Source: three-view drawing plus pictorial views. Frame: mm from the lowest corner of the part. A direction names the side the tool comes from. Round coordinates to 2 decimals unless told otherwise and drop trailing zeros. Write each loop counter-clockwise with the first axis right and the second up, starting at its lowest first coordinate (ties: lowest second). Pieces come first, ordered by that corner, then holes. Notation, with made-up numbers: (64, 75) -> (101, 75) arc R7 cw to (101, 82) -> close; hole circle Ø10 at (69, -3.75). An arc over 180 degrees is marked (long way). Put each result on its own line as item: value.
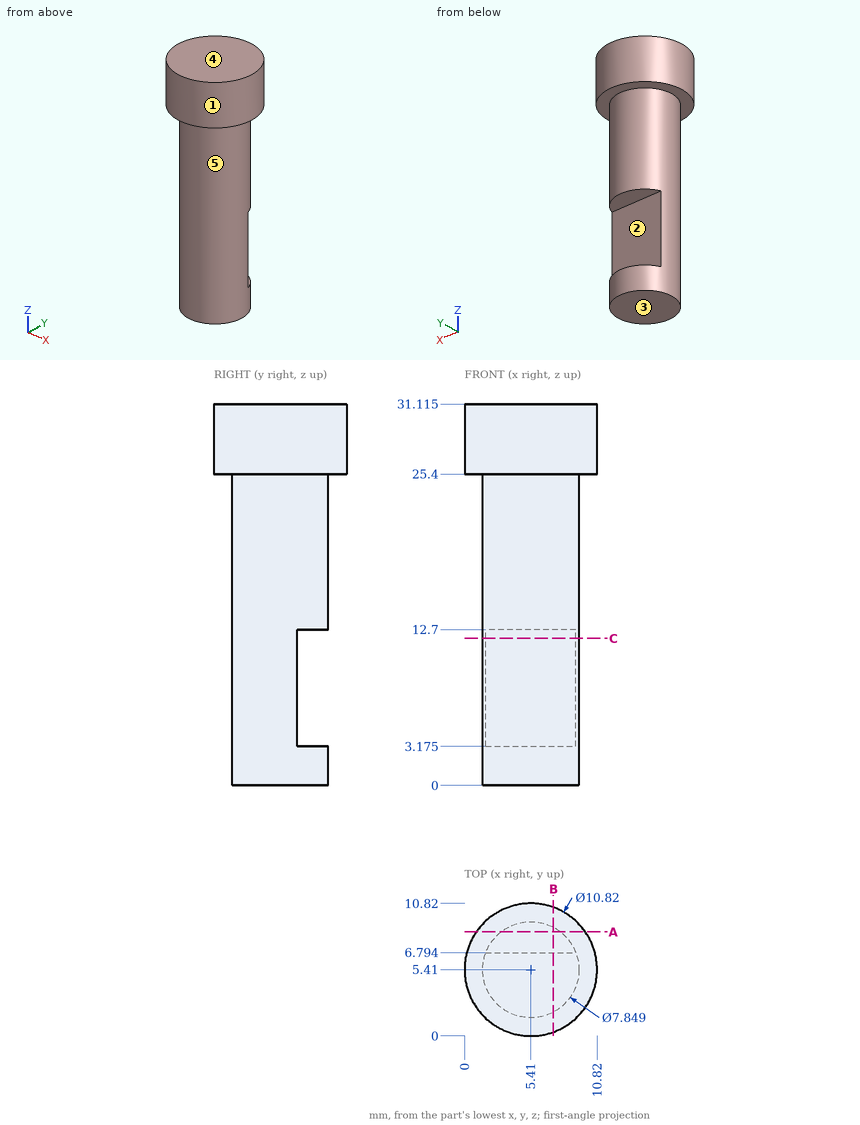
Q1. Cut plane C-C on z = 12. Output: boundary loops of the cut face in (x, y) (1 decimal), and give its area (3 significant figures).
Ans:
outline: (1.7, 6.8) arc R3.9 ccw (long way) to (9.1, 6.8) -> close
area: 34.8 mm^2
Q2. Reachability of the marked faces 4 and 5 from +Z, -Z, +X, -X, +Y, -Y: full face, straight path, thin tool, end or side. Return the list, or none.
Ans:
face 4: +Z, +X, -X, +Y, -Y
face 5: -Z
Q3. Pin query (flat end, axial travel): pin 1 (1 mm diameter, centred on x = 6.5, y = 2, fed in from -Z); pin 2 (2 mm diameter, centred on x = 6, z = 9, fed in from +Y) (1 decimal); pin 3 (2 mm diameter, centred on x = 2.5, z = 12.5, fed in from +Y); pin 4 (3 mm diameter, centred on y = 3, z = 22.5, fed in from +X). Return the tip coordinate at first contact, or that it passes through.
Ans:
pin 1: stops at z = 0
pin 2: stops at y = 6.8
pin 3: stops at y = 8.83
pin 4: stops at x = 9.23
Q4. Material intervals for line 1 (Z direction, x = 7.5, y = 7.5) (1 decimal); line 2 (Z direction, x = 10, y = 6.25) (1 decimal); line 3 (X direction, y = 5.25, z = 18), sorted ascending. Write a range as [from, to].
Ans:
line 1: z = [0, 3.2], [12.7, 31.1]
line 2: z = [25.4, 31.1]
line 3: x = [1.49, 9.33]
Q5. Cut plane B-B on x = 7.25. Output: boundary loops of the cut face in (y, z) (1 decimal), and give its area (3 significant figures).
Ans:
outline: (0.3, 25.4) -> (1.9, 25.4) -> (1.9, 0) -> (8.9, 0) -> (8.9, 3.2) -> (6.8, 3.2) -> (6.8, 12.7) -> (8.9, 12.7) -> (8.9, 25.4) -> (10.5, 25.4) -> (10.5, 31.1) -> (0.3, 31.1) -> close
area: 214 mm^2
Q6. Draft query along Z for the marked faces 1, 2 and 3. Return one class per face: +Z half, -Z half, draft (parallel to the pull), parting line (faces both ways), or undercut.
Ans:
face 1: draft
face 2: undercut
face 3: -Z half
Q7. Cut plane A-A on y = 8.5. Output: boundary loops of the cut face in (x, z) (1 decimal).
Ans:
outline: (1, 25.4) -> (3, 25.4) -> (3, 12.7) -> (7.8, 12.7) -> (7.8, 25.4) -> (9.9, 25.4) -> (9.9, 31.1) -> (1, 31.1) -> close; (3, 0) -> (7.8, 0) -> (7.8, 3.2) -> (3, 3.2) -> close
